```python
from build123d import *

# Parameters (mm, degrees)
BOSS_EXTRUDE1_DEPTH = 3.175
CUT_EXTRUDE1_DEPTH  = 3.175
FILLET4_R           = 2.54
FILLET5_R           = 2.54


with BuildPart() as part:
    # Sketch1 → Boss-Extrude1 (new body)
    with BuildSketch(Plane.XY):
        Polygon((0, 0), (0, 50.8), (3.175, 50.8), (50.8, 3.175), (50.8, 0), align=None)
    extrude(amount=BOSS_EXTRUDE1_DEPTH)

    # Sketch7 → Cut-Extrude1 (cut)
    with BuildSketch(Plane.XY.offset(3.175)):
        Polygon((6.35, 41.275), (6.35, 6.35), (41.275, 6.35), align=None)
    extrude(amount=-CUT_EXTRUDE1_DEPTH, mode=Mode.SUBTRACT)

    # Fillet4
    fillet4_edges = [part.edges().sort_by_distance(p)[0] for p in [
        (50.8, 3.175, 1.5875),
        (3.175, 50.8, 1.5875),
    ]]
    fillet(fillet4_edges, radius=FILLET4_R)

    # Fillet5
    fillet5_edges = [part.edges().sort_by_distance(p)[0] for p in [
        (6.35, 6.35, 1.5875),
        (41.275, 6.35, 1.5875),
        (6.35, 41.275, 1.5875),
    ]]
    fillet(fillet5_edges, radius=FILLET5_R)


solid = part.part
```
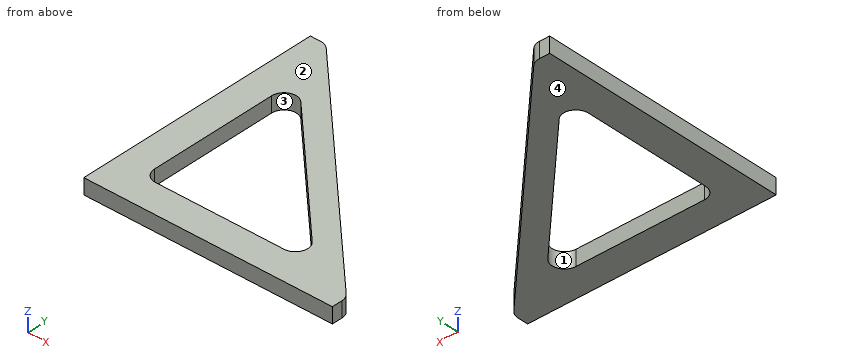
Could you check a few things on this model? Use its own coordinates, in mm. Face numbers are marked on the shaded views. A direction names the side the tool comes from. Coordinates: 2 decimals unless noted, no trailing zeros. Loops run counter-clockwise (first coordinate to the right, second up) from the corner with the lowest first, then second, coordinate; pieces in that order, holes last.
1) Will these pins go through, and if not, where does the flat tip stop? pin 1 Ø1 at (y, z) = (16, 2) entering from +X (3 decimals); pin 2 Ø1.6 at (x, z) = (27, 1.5) entering from +Y (3 decimals).
Reported:
pin 1: stops at x = 38.475
pin 2: stops at y = 27.775
2) Please list where these lines run through material, in increasing order: line 1 along Y through (x, z) = (23, 2) (3 decimals); line 2 along Y through (x, z) = (35, 0.75) (3 decimals); line 3 along X through (y, z) = (7.5, 1.15) (3 decimals).
Reported:
line 1: y = 0 to 6.35, 24.625 to 30.975
line 2: y = 0 to 6.35, 12.625 to 18.975
line 3: x = 0 to 6.764, 37.269 to 46.475
3) Which directions (+Z, -Z, +X, -X, +Y, -Y) give clear straight access to the entire face, cutting with the end or side of a thin tool? Please do the marked faces 3 and 4.
Reported:
face 3: +Z, -Z
face 4: -Z, +X, -X, +Y, -Y
4) Imagine slicing it at D-D (y = 47). List the corners of the cut face in (x, z) for me (3 decimals).
Reported:
outline: (0, 0) - (6.975, 0) - (6.975, 3.175) - (0, 3.175) - close
5) Thinking about a two-plate mould opening in X: for the marked faces 1 and 2, which applies, released by +X, released by -X, zero draft, split by the parting line, or undercut?
Reported:
face 1: undercut
face 2: zero draft
6) Imagine slicing it at A-A (y = 13.5). List the corners of the cut face in (x, z) for me (3 decimals).
Reported:
outline: (0, 0) - (6.35, 0) - (6.35, 3.175) - (0, 3.175) - close; (34.125, 0) - (40.475, 0) - (40.475, 3.175) - (34.125, 3.175) - close
7) Imagine slicing it at C-C (x = 27). List the corners of the cut face in (y, z) for me (3 decimals).
Reported:
outline: (0, 0) - (6.35, 0) - (6.35, 3.175) - (0, 3.175) - close; (20.625, 0) - (26.975, 0) - (26.975, 3.175) - (20.625, 3.175) - close
8) Imagine slicing it at B-B (z = 0.5). List the corners of the cut face in (x, y) for me.
Reported:
outline: (0, 0) - (50.8, 0) - (50.8, 2.12) arc R2.54 ccw to (50.06, 3.92) - (3.92, 50.06) arc R2.54 ccw to (2.12, 50.8) - (0, 50.8) - close; hole (6.35, 8.89) arc R2.54 ccw to (8.89, 6.35) - (35.14, 6.35) arc R2.54 ccw to (36.94, 10.69) - (10.69, 36.94) arc R2.54 ccw to (6.35, 35.14) - close
